from build123d import *

# Parameters (mm, degrees)
F0_W     = 15.24
F0_H     = 38.1
F1_DEPTH = 1.27
F5_D     = 1.524
F6_R     = 1.016
F7_DEPTH = 15.241


# Not quite as in the source:
# - the program builds the solid bodies; features that only make, move or delete a surface that nothing else refers to are left out


with BuildPart() as f1:
    # F0 (on Front) → F1 (new body, symmetric)
    with BuildSketch(Plane.XZ):
        Rectangle(F0_W, F0_H)
    extrude(amount=F1_DEPTH, both=True)

    # F5 (through all)
    with Locations(Plane.YZ.offset(7.62)):
        with Locations((0, 14.5949712023)):
            Hole(F5_D / 2)

    # F6 (on face) → F7 (cut, through all)
    with BuildSketch(Plane.YZ.offset(7.62)):
        with Locations((0, 7.4023683179)):
            Circle(F6_R)
    extrude(amount=-F7_DEPTH, mode=Mode.SUBTRACT)


solid = f1.part
Work out the finished part from the listing and answer in its coordinate system (mm). Round coordinates to 2 decimals unless told otherwise and drop trailing zeros. Write each loop counter-clockwise with the first axis right and the second up, starting at its lowest first coordinate (ties: lowest second). Pieces come first, ordered by that corner, then holes. Notation, with made-up numbers: (45, 39) -> (66, 39) arc R23 ccw to (66, 48) -> close; hole circle Ø10 at (5, -14). An arc over 180 degrees is marked (long way). Answer as CSV lines item,"result". Start each with the question number.
(1) The part is cut by section B-B, the plane x = -2.25. Give the vertices of the cut face in (y, z).
(2) Find the intervals of material crossed by probe 1 along Z at (x, y) = (4.25, 0); probe 2 along Z at (x, y) = (1.75, 0.45); probe 3 along Z at (x, y) = (2.5, -0.8), in increasing order.
(3) The part is cut by section A-A, the plane y = 0. Give the vertices of the cut face in (x, z), then the cut area to 3 significant figures.
(4) The mould has two halves that part along Y. Classify faces 1 (the flat face through (0, 1.27, 0)), 2 (the cylindrical face through (0.11, -0.13, 8.41)), 3 (the flat face through (7.62, 0, 0)): +Y half, -Y half, draft (parallel to the pull), parting line (faces both ways), or undercut.
Output values:
1,outline,"(-1.27, -19.05) -> (1.27, -19.05) -> (1.27, 19.05) -> (-1.27, 19.05) -> close; hole circle Ø2.03 at (0, 7.4); hole circle Ø1.52 at (0, 14.59)"
2,probe 1,"z = -19.05 to 6.39, 8.42 to 13.83, 15.36 to 19.05"
2,probe 2,"z = -19.05 to 6.49, 8.31 to 13.98, 15.21 to 19.05"
2,probe 3,"z = -19.05 to 6.78, 8.03 to 19.05"
3,outline,"(-7.62, -19.05) -> (7.62, -19.05) -> (7.62, 6.39) -> (-7.62, 6.39) -> close; (-7.62, 8.42) -> (7.62, 8.42) -> (7.62, 13.83) -> (-7.62, 13.83) -> close; (-7.62, 15.36) -> (7.62, 15.36) -> (7.62, 19.05) -> (-7.62, 19.05) -> close"
3,area,"526 mm²"
4,face 1,"+Y half"
4,face 2,"undercut"
4,face 3,"draft"
